Geometry check sheet. Reference: the model listing, model coordinates, mm. A direction names the side the tool comes from. Round coordinates to 2 decimals unless told otherwise and drop trailing zeros. Order: outer loops, then holes, each group sorted by start corner. A loop starts at its lowest first (then second) coordinate and runs counter-clockwise, first axis right, second up.
(1) Set-up check for faces 4 (the face through (-31.182, 3, -15)), 5 (the face through (-57, 3, -126.861)), 6 (the face through (-22, 3, -136.861)): record each of +Z, -Z, +X, -X, +Y, -Y from which the full face is reachable in a straight line by a thin tool's end or side.
(2) Cross-section at A-A on y = 1.6. Enter the section's corners in (x, z), and give its area (3 significant figures).
(3) Cross-section at B-B on x = -6.5. Enter the section's corners in (y, z).
(4) Draft check along X on faces 1 (the face through (-53.514, 3, -133)), 2 (the face through (-37, 3, -17.361)), 3 (the face through (-137.42, 2.96, -83.88)). Enter one of: pulls with the +X half, pulls with the -X half, needs draft (parallel to the pull), parting line crosses it, or undercut.
(5) Cross-section at C-C on z = -27. Enter the section's corners in (x, y).
(6) Gauge pin test, flat ends, axial feed: P1, Ø3.5, axis at y = 2.5, z = -15.5, coming from the +X side; P2, Ø1.8, axis at y = 4.5, z = -29, coming from the -X side; P3, Ø3, axis at y = 1.5, z = -132, coming from the -X side. Record the tip position at first contact, or that the pin passes through.
(7) Thickness scan on L1, parallel to Z at x = -48, y = 4.45; L2, parallel to Z at x = -58.5, y = 3.15; L3, parallel to X at y = 2.85, z = -20. Record the ranges inside material, lowest first.
Autodesk Inventor part; units mm, degrees
ref_plane "YZ Plane" through (0, 0, 0) normal (1, 0, 0) x (0, 1, 0)
ref_plane "XZ Plane" through (0, 0, 0) normal (0, 1, 0) x (-1, 0, 0)
ref_plane "XY Plane" through (0, 0, 0) normal (0, 0, 1) x (1, 0, 0)
sketch "Sketch1" plane through (0, 0, 0) normal (0, 1, 0) x (-1, 0, 0)
  arc A0 (-1.4864, -17.3614) -> (1.1787, -17.296) centre (-0.1546, -17.296) ccw
  arc A1 (31.1823, -17.2881) -> (33.847, -17.3614) centre (32.5157, -17.2881) ccw
  line L0 (33.847, -17.3614) -> (41.1803, -17.3614)
  line L1 (-1.4864, -17.3614) -> (-8.8197, -17.3614)
  line L2 (-8.8197, -17.3614) -> (-8.8197, -136.8614)
  line L3 (41.1803, -17.3614) -> (41.1803, -38.0281)
  arc A2 (41.1803, -38.0281) -> (40.0555, -40.0773) centre (40.0555, -38.7439) ccw
  line L4 (40.0555, -40.0773) -> (85.8888, -40.0773)
  line L5 (-8.8197, -136.8614) -> (53.5136, -136.8614)
  line L6 (53.5136, -136.8614) -> (53.5136, -129.5281)
  arc A3 (53.5136, -126.8614) -> (53.5136, -129.5281) centre (53.5136, -128.1947) ccw
  arc A4 (60.0136, -129.5281) -> (60.0136, -126.8614) centre (60.0136, -128.1947) ccw
  line L7 (60.0136, -129.5281) -> (60.0136, -142.8614)
  line L8 (60.0136, -126.8614) -> (53.5136, -126.8614)
  line L9 (120.137, -136.8614) -> (120.137, -129.5281)
  arc A5 (120.137, -129.5281) -> (120.137, -126.8614) centre (120.137, -128.1947) ccw
  arc A6 (113.637, -126.8614) -> (113.637, -129.5281) centre (113.637, -128.1947) ccw
  line L10 (113.637, -129.5281) -> (113.637, -142.8614)
  line L11 (113.637, -126.8614) -> (120.137, -126.8614)
  arc A7 (182.4703, -136.8614) -> (85.8888, -40.0773) centre (-162.7379, -384.7652) ccw
  line L12 (120.137, -136.8614) -> (182.4703, -136.8614)
  arc A8 (2.512, -11.3614) -> (1.1787, -12.6947) centre (2.512, -12.6947) ccw
  line L13 (1.1787, -12.6947) -> (1.1787, -17.296)
  arc A9 (31.1823, -12.6947) -> (29.849, -11.3614) centre (29.849, -12.6947) ccw
  line L14 (2.512, -11.3614) -> (29.849, -11.3614)
  line L15 (31.1823, -17.2881) -> (31.1823, -12.6947)
  line L16 (60.0136, -142.8614) -> (113.637, -142.8614)
  point P0 (0, 0)
  point P1 (28.8512, 3.0303)
  point P2 (-1.1488, 3.0309)
  dimension "d1" = 2.6667
  dimension "d2" = 30
  dimension "d4" = 2.6667
  dimension "d6" = 7.3333
  dimension "d7" = 7.3333
  dimension "d8" = 20.6667
  dimension "d9" = 2.6667
  dimension "d10" = 45.8333
  dimension "d11" = 119.5
  dimension "d12" = 62.3333
  dimension "d19" = 7.3333
  dimension "d53" = 2.6667
  dimension "d56" = 2.6667
  dimension "d58" = 6.5
  dimension "d59" = 13.3333
  dimension "d61" = 425
  dimension "d64" = 13.3333
  dimension "d67" = 7.3333
  dimension "d73" = 50
  dimension "d74" = 2.6667
  dimension "d75" = 6
  dimension "d76" = 191.29
  dimension "d77" = 6.5
  dimension "d78" = 6.5
  dimension "d79" = 6.5
  dimension "d80" = 1.3333
  dimension "d81" = 1.3333
  dimension "d82" = 90
  dimension "d83" = 2.6667
  dimension "d84" = 2.6667
  dimension "d85" = 2.6667
  dimension "d86" = 2.6667
  dimension "d87" = 53.6233
extrude "Extrusion1" add sketch "Sketch1" along normal blind 6
properties part number "Support A1" material "Wood (Maple)"
Found:
1. face 4: +Z, -X, +Y, -Y
1. face 5: -Z, +Y, -Y
1. face 6: -Z, +X, +Y, -Y
2. outline: (-182.47, -136.86) - (-120.14, -136.86) - (-120.14, -129.53) arc R1.33 cw to (-120.14, -126.86) - (-113.64, -126.86) arc R1.33 cw to (-113.64, -129.53) - (-113.64, -142.86) - (-60.01, -142.86) - (-60.01, -129.53) arc R1.33 cw to (-60.01, -126.86) - (-53.51, -126.86) arc R1.33 cw to (-53.51, -129.53) - (-53.51, -136.86) - (8.82, -136.86) - (8.82, -17.36) - (1.49, -17.36) arc R1.33 cw to (-1.18, -17.3) - (-1.18, -12.69) arc R1.33 ccw to (-2.51, -11.36) - (-29.85, -11.36) arc R1.33 ccw to (-31.18, -12.69) - (-31.18, -17.29) arc R1.33 cw to (-33.85, -17.36) - (-41.18, -17.36) - (-41.18, -38.03) arc R1.33 cw (long way) to (-40.06, -40.08) - (-85.89, -40.08) arc R425 ccw to start
2. area: 15,800 mm2
3. outline: (0, -136.86) - (6, -136.86) - (6, -11.36) - (0, -11.36) - close
4. face 1: undercut
4. face 2: needs draft
4. face 3: pulls with the -X half
5. outline: (-41.18, 0) - (8.82, 0) - (8.82, 6) - (-41.18, 6) - close
6. P1: stops at x = -1.18
6. P2: stops at x = -41.18
6. P3: stops at x = -180.03
7. L1: z = -136.86 to -40.08
7. L2: z = -126.86 to -40.08
7. L3: x = -41.18 to 8.82
